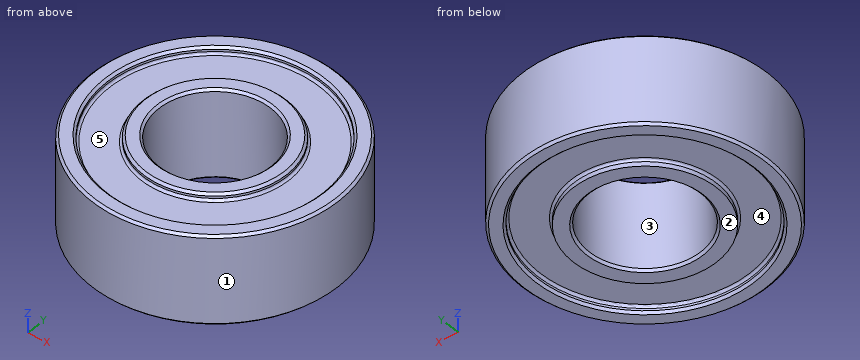
Autodesk Inventor part; units mm, degrees
ref_plane "Work Plane1" through (0, 0, 2) normal (0, 0, 1) x (1, 0, 0)
ref_plane "YZ Plane" through (0, 0, 0) normal (1, 0, 0) x (0, 1, 0)
ref_plane "XZ Plane" through (0, 0, 0) normal (0, 1, 0) x (-1, 0, 0)
sketch "Sketch1" plane through (0, 0, 0) normal (0, 0, 1) x (1, 0, 0)
  circle A0 centre (0, 0) radius 5.5
  dimension "d0" = 11
extrude "Extrusion1" add sketch "Sketch1" along normal blind 4
sketch "Sketch2" plane through (0, 0, 4) normal (0, 0, 1) x (1, 0, 0)
  circle A0 centre (0, 0) radius 2.5
  dimension "d3" = 5
extrude "Extrusion2" cut sketch "Sketch2" against normal through all
sketch "Sketch3" plane through (0, 0, 4) normal (0, 0, 1) x (1, 0, 0)
  circle A0 centre (0, 0) radius 3.2
  circle A1 centre (0, 0) radius 4.8
  circle A2 centre (0, 0) radius 2.5
  circle A3 centre (0, 0) radius 5.5
  dimension "d6" = 0.7
  dimension "d7" = 0.7
extrude "Extrusion3" cut sketch "Sketch3" against normal blind 0.3 contours A1
chamfer "Chamfer1" distance 0.1 angle 45 4 edges at (-4.8, 0, 4) (-5.5, 0, 4) (-3.2, 0, 4) (-2.5, 0, 4)
fillet "Fillet1" radius 0.1 2 edges at (-4.8, 0, 3.7) (-3.2, 0, 3.7)
ref_plane "Work Plane1" through (0, 0, 2) normal (0, 0, 1) x (1, 0, 0)
mirror "Mirror1" about plane through (0, 0, 2) normal (0, 0, 1) of "Extrusion3", "Fillet1"
chamfer "Chamfer2" distance 0.1 angle 45 3 edges at (-5.5, 0, 0) (-4.8, 0, 0) (-2.5, 0, 0)
properties part number "MR115 2RS" material "Steel, Alloy"
Build history of the part. All positions in model axes, mm. Face numbers are marked on the shaded views. A direction names the side the tool comes from. Round coordinates to 2 decimals unless told otherwise and drop trailing zeros. Write each loop counter-clockwise with the first axis right and the second up, starting at its lowest first coordinate (ties: lowest second). Pieces come first, ordered by that corner, then holes. Notation, with made-up numbers: M -5,-10 L 0,-10 A5 cw 0,-1 Z; hole C 31.5,62 d10. An arc over 180 degrees is marked long. Answer in a Markdown table with one row per item.
1. Saw through at A-A (z = 1.5). List the corners of the cut face in (x, y).
Geometry check:
| item | result |
|---|---|
| outline | C 0,0 d11; hole C 0,0 d5 |
2. Probe L1, parallel to Y at x = 0, z = 1.9; L2, parallel to Z at x = -3.25, y = 1.25; L3, parallel to X at y = 1.5, z = 2.3. List the from-to ranges inside material, lowest first. Write a range as [from, to].
Geometry check:
| item | result |
|---|---|
| L1 | [-5.5, -2.5], [2.5, 5.5] |
| L2 | [0.3, 3.7] |
| L3 | [-5.29, -2], [2, 5.29] |
3. Flat gauge pins, fed straight in: P1, Ø1.5, axis at y = -3, z = 2.5, coming from the +X side; P2, Ø1, axis at x = 1, z = 2, coming from the -Y side. Where does each tip first touch, or does it go through?
Geometry check:
| item | result |
|---|---|
| P1 | x = 5.02 |
| P2 | y = -5.48 |
4. Which spindle directions (+Z, -Z, +X, -X, +Y, -Y) get a long thin tool onto all of the face, cutting with end or side? Do the marked faces 4 and 5. Say none if no direction does.
Geometry check:
| item | result |
|---|---|
| face 4 | -Z |
| face 5 | +Z |
5. Mould opens along Y. For the marked faces 1, 2 and 3 say: +Y half, -Y half, draft (parallel to the pull), parting line (faces both ways), or undercut.
Geometry check:
| item | result |
|---|---|
| face 1 | parting line |
| face 2 | draft |
| face 3 | undercut |
